Work out the finished part from the listing and answer in its coordinate system (mm). A direction names the side the tool comes from. Give positions to 0.01 mm unless a question says otherwise; leave off trailing zeros. Order: outer loops, then holes, each group sorted by start corner. A loop starts at its lowest first (then second) coordinate and runs counter-clockwise, first axis right, second up. Notation, with made-up numbers: (28, 87) - (81, 87) arc R13 ccw to (81, 109) - close; hole circle Ø9 at (-29, -7). An arc over 180 degrees is marked (long way). Put each result on its own line as item: value.
```python
from build123d import *

# Parameters (mm, degrees)
F0_W     = 203.2
F0_H     = 203.2
F0_W_2   = 165.1
F0_H_2   = 165.1
F1_DEPTH = 254
F2_DEPTH = 19.05
F3_R     = 17.78
F4_DEPTH = 25.4


with BuildPart() as f1:
    # F0 (on Top) → F1 (new body)
    with BuildSketch(Plane.XY):
        with Locations((-14.190134, 8.51027)):
            Rectangle(F0_W, F0_H)
        with Locations((-14.190134, 8.51027)):
            Rectangle(F0_W_2, F0_H_2, mode=Mode.SUBTRACT)
    extrude(amount=-F1_DEPTH)

    # F0 (on Top) → F2 (join)
    with BuildSketch(Plane.XY):
        with Locations((-14.190134, 8.51027)):
            Rectangle(F0_W_2, F0_H_2)
    extrude(amount=-F2_DEPTH)

    # F3 (on face) → F4 (cut)
    with BuildSketch(Plane(origin=(-115.790134, 0, 0), x_dir=(0, -1, 0), z_dir=(-1, 0, 0))):
        with Locations((0, -205.345541)):
            Circle(F3_R)
    extrude(amount=-F4_DEPTH, mode=Mode.SUBTRACT)


solid = f1.part
```
(1) Section D-D, the plane y = 50 is taken. Write down the section's boundary in (x, z).
Geometry check:
outline: (-115.79, -254) - (-96.74, -254) - (-96.74, -19.05) - (68.36, -19.05) - (68.36, -254) - (87.41, -254) - (87.41, 0) - (-115.79, 0) - close
(2) Section A-A, the plane y = 0 is taken. Write down the section's boundary in (x, z), then the cut area to 3 significant figures.
Geometry check:
outline: (-115.79, -254) - (-96.74, -254) - (-96.74, -223.13) - (-115.79, -223.13) - close; (-115.79, -187.57) - (-96.74, -187.57) - (-96.74, -19.05) - (68.36, -19.05) - (68.36, -254) - (87.41, -254) - (87.41, 0) - (-115.79, 0) - close
area: 12,100 mm²
(3) A tool of negligible diameter and unlimited length cuts with its end or side. For faces 5 (the face through (-15, -74.04, -135)), 6 (the face through (-16, -93.09, -125)), 7 (the face through (-106.4, -8.2, -221.12)), from which of +Z, -Z, +X, -X, +Y, -Y can it reach the whole face along a straight path? Write none if from no direction.
Geometry check:
face 5: -Z
face 6: +Z, -Z, +X, -X, -Y
face 7: -X
(4) Section C-C, the plane x = -67 is taken. Write down the section's boundary in (y, z).
Geometry check:
outline: (-93.09, -254) - (-74.04, -254) - (-74.04, -19.05) - (91.06, -19.05) - (91.06, -254) - (110.11, -254) - (110.11, 0) - (-93.09, 0) - close
(5) Section B-B, the plane z = -174.5 is taken. Write down the section's boundary in (x, y), then the cut area to 3 significant figures.
Geometry check:
outline: (-115.79, -93.09) - (87.41, -93.09) - (87.41, 110.11) - (-115.79, 110.11) - close; hole (-96.74, -74.04) - (68.36, -74.04) - (68.36, 91.06) - (-96.74, 91.06) - close
area: 14,000 mm²
(6) Given pin 1 (1 mm diameter, centred on x = 19.5, y = 49, fed in from -Z), flat-ended and moving along its own axis, determine where the tip first touches the part or whether it passes through.
Geometry check:
pin 1: stops at z = -19.05
(7) Straight lines are drawn through the part: line 1 (Y direction, x = -71.5, z = -118.5); line 2 (X direction, y = 41, z = -237.5); line 3 (Z direction, x = -105, y = 0). For each, find the intervals that lie inside material, in ascending order.
Geometry check:
line 1: y = -93.09 to -74.04, 91.06 to 110.11
line 2: x = -115.79 to -96.74, 68.36 to 87.41
line 3: z = -254 to -223.13, -187.57 to 0
(8) Determine the mould class of faces 1 (the face through (-16, 110.11, -125)), 2 (the face through (-16, 10, 0)), 3 (the face through (-15, 91.06, -135)), 4 (the face through (-15, 10, -19.05)) for opening direction Y: pulls with the +Y half, pulls with the -Y half, needs draft (parallel to the pull), parting line crosses it, or undercut.
Geometry check:
face 1: pulls with the +Y half
face 2: needs draft
face 3: undercut
face 4: undercut
